Geometry: final body of the model. Coordinates: model frame, mm. A direction names the side the tool comes from. Round coordinates to 2 decimals unless told otherwise and drop trailing zeros. Order: outer loops, then holes, each group sorted by start corner. A loop starts at its lowest first (then second) coordinate and runs counter-clockwise, first axis right, second up. Notation, with made-up numbers: (-26, 5.5) - (28, 5.5) arc R24 ccw to (28, 20.5) - close; hole circle Ø3 at (30, 80.5). An arc over 180 degrees is marked (long way). Put each result on its own line as item: value. Start each with the question number.
(1) Material intervals for L1, parallel to Y at x = 3.25, z = -5.75; L2, parallel to X at y = 92, z = -4; L3, parallel to X at y = 37, z = -6.25, sorted ascending. Write a range as [from, to].
(2) Pull-direction query (Y, two-part tool) for faces 1 (the face through (3.397, 90.088, -3.757)), 2 (the face through (3.81, 30, -4)), 3 (the face through (0.76, 103.92, -3.86)), 4 (the face through (-3.563, 2.504, -5.692)); classes: released by +Y, released by -Y, zero draft, split by the parting line, or undercut.
(3) Section C-C (y = 85). Output: boundary loops of the cut face in (x, z).
(4) Access query for faces 5 (the face through (10, 102.108, -4)), 6 (the face through (-1, 5.08, -4)), 7 (the face through (0, 81, -4)). Directions: +Z, -Z, +X, -X, +Y, -Y. A direction counts if a zero-diameter tool reaches every point of the face in a straight line with its end or side. Return the directions, or none.
(5) Section D-D (x = 9). Output: boundary loops of the cut face in (y, z).
(6) Pin query (flat end, axial travel): P1, Ø3, axis at x = 10, z = -3.5, coming from the -Y side; P2, Ø4, axis at x = -1.5, z = -4, coming from the +Y side; P3, Ø2, axis at x = 1, z = -1.5, coming from the +Y side. Return the tip coordinate at first contact, or that it passes through.
(7) Section A-A (x = -3.81). Output: boundary loops of the cut face in (y, z).
(8) Section B-B (z = -3.81). Output: boundary loops of the cut face in (x, y) (3 decimals).
from build123d import *

# Parameters (mm, degrees)
SKETCH1_W             = 7.62
SKETCH1_H             = 104.648
BOSS_EXTRUDE1_DEPTH   = 7.62
SKETCH2_W             = 7.62
SKETCH2_H             = 5.08
BOSS_EXTRUDE2_DEPTH   = 7.62
SKETCH4_W             = 7.62
SKETCH4_H             = 2.54
BOSS_EXTRUDE3_DEPTH   = 8.128
BOSS_EXTRUDE4_DEPTH   = 2.54
F_6_CLEARANCE_HOLE1_D = 3.7973
CUT_EXTRUDE1_DEPTH    = 2.54
SKETCH12_W            = 7.62
SKETCH12_H            = 45.72
CUT_EXTRUDE2_DEPTH    = 3.81
FILLET2_R             = 12.7
FILLET3_R             = 2.54
SKETCH14_R            = 1.905
CUT_EXTRUDE4_DEPTH    = 107.100272422


with BuildPart() as part:
    # Sketch1 → Boss-Extrude1 (new body)
    with BuildSketch(Plane(origin=(0, 0, 0), x_dir=(0, 0, -1), z_dir=(1, 0, 0))):
        with Locations((3.81, 52.324)):
            Rectangle(SKETCH1_W, SKETCH1_H)
    extrude(amount=BOSS_EXTRUDE1_DEPTH)

    # Sketch2 → Boss-Extrude2 (add)
    with BuildSketch(Plane.ZY):
        with Locations((-3.81, 2.54)):
            Rectangle(SKETCH2_W, SKETCH2_H)
    extrude(amount=BOSS_EXTRUDE2_DEPTH)

    # Sketch4 → Boss-Extrude3 (add)
    with BuildSketch(Plane(origin=(7.62, 0, 0), x_dir=(0, 0, -1), z_dir=(1, 0, 0))):
        with Locations((3.81, 103.378)):
            Rectangle(SKETCH4_W, SKETCH4_H)
    extrude(amount=BOSS_EXTRUDE3_DEPTH)

    # Sketch5 → Boss-Extrude4 (add)
    with BuildSketch(Plane.XZ.offset(-102.108)):
        Polygon((15.748, 0), (12.974546815, -7.62), (10.434546815, -7.62), (13.208, 0), align=None)
    extrude(amount=BOSS_EXTRUDE4_DEPTH)

    # #6 Clearance Hole1 (through all)
    with Locations(Plane(origin=(0, 5.08, 0), x_dir=(1, 0, 0), z_dir=(0, 1, 0))):
        with Locations((-3.81, 3.81)):
            Hole(F_6_CLEARANCE_HOLE1_D / 2)

    # Sketch8 → Cut-Extrude1 (cut)
    with BuildSketch(Plane.XZ.offset(-102.108)):
        Polygon((15.748, -7.62), (12.974546815, -7.62), (15.748, 0), align=None)
    extrude(amount=-CUT_EXTRUDE1_DEPTH, mode=Mode.SUBTRACT)

    # Sketch12 → Cut-Extrude2 (cut)
    with BuildSketch(Plane.ZY):
        with Locations((-3.81, 27.94)):
            Rectangle(SKETCH12_W, SKETCH12_H)
    extrude(amount=-CUT_EXTRUDE2_DEPTH, mode=Mode.SUBTRACT)

    # Fillet2
    # the kernel refuses this fillet: 12.7 mm, written as the material it takes off along each edge
    with BuildSketch(Plane(origin=(0, 50.8, 22.674035261), x_dir=(1, 0, 0), z_dir=(0, 0, -1))) as fillet2_piece_1:
        with BuildLine():
            CenterArc((12.7, -9.069614104), FILLET2_R, 134.427004001, 45.572995999)
            Line((0, -9.069614104), (-0.254, -9.069614104))
            Line((-0.254, -9.069614104), (-0.254, 0))
            Line((-0.254, 0), (0, 0.254))
            ThreePointArc((0, 0.254), (1.905, 0.254), (3.6322, 0.181392282))
            Line((3.6322, 0.181392282), (3.81, 0))
        make_face()
    extrude(amount=52.968070521, mode=Mode.SUBTRACT)

    # Fillet3
    fillet3_edges = [part.edges().sort_by_distance(p)[0] for p in [
        (3.81, 5.08, -3.81),
        (7.62, 0, -3.81),
        (0, 104.648, -3.81),
    ]]
    fillet(fillet3_edges, radius=FILLET3_R)

    # Sketch14 → Cut-Extrude4 (cut, through all)
    with BuildSketch(Plane.XY):
        with Locations((3.81, 91.948)):
            Circle(SKETCH14_R)
        with Locations((3.81, 81.788)):
            Circle(SKETCH14_R)
    extrude(amount=-CUT_EXTRUDE4_DEPTH, mode=Mode.SUBTRACT)


solid = part.part
Checks:
1. L1: y = [0, 6.03], [51.39, 79.97], [83.61, 90.13], [93.77, 104.65]
1. L2: x = [0, 1.91], [5.71, 7.62]
1. L3: x = [3.81, 7.62]
2. face 1: undercut
2. face 2: undercut
2. face 3: released by +Y
2. face 4: zero draft
3. outline: (0, -7.62) - (7.62, -7.62) - (7.62, 0) - (0, 0) - close
4. face 5: +Z, -Y
4. face 6: +Z, -Z, -X
4. face 7: +Z, -Z, -X, +Y
5. outline: (102.11, -7.62) - (104.65, -7.62) - (104.65, 0) - (102.11, 0) - close
6. P1: stops at y = 102.11
6. P2: stops at y = 103.62
6. P3: stops at y = 104.59
7. outline: (0, -7.62) - (5.08, -7.62) - (5.08, -5.71) - (0, -5.71) - close; (0, -1.91) - (5.08, -1.91) - (5.08, 0) - (0, 0) - close
8. outline: (-7.62, 0) - (-5.709, 0) - (-5.709, 5.08) - (-7.62, 5.08) - close; (-1.911, 0) - (5.08, 0) arc R2.54 ccw to (7.62, 2.54) - (7.62, 102.108) - (11.821, 102.108) - (11.821, 99.568) - (14.361, 99.568) - (14.361, 104.648) - (2.54, 104.648) arc R2.54 ccw to (0, 102.108) - (0, 59.87) arc R12.7 ccw to (3.81, 50.8) - (3.81, 7.62) arc R2.54 cw to (1.27, 5.08) - (-1.911, 5.08) - close; hole circle Ø3.81 at (3.81, 81.788); hole circle Ø3.81 at (3.81, 91.948)
